Geometry: final body of the model. Coordinates: model frame, mm. Face numbers are marked on the shaded views. A direction names the side the tool comes from. Give positions to 0.01 mm unless a question says otherwise; leave off trailing zeros. Loops run counter-clockwise (first coordinate to the right, second up) from the corner with the lowest first, then second, coordinate; pieces in that order, holes last. Notation, with made-up numbers: (-36, 51) -> (-22, 51) arc R12 cw to (-22, 62) -> close; hole circle Ø1 at (-23, 46). An arc over 180 degrees is marked (long way). Answer in a Markdown table with one row per item. Add a question column.
1) Section query C-C (z = -4.5). Return the cut outline in (x, y) (3 decimals), plus the area to 3 significant figures.
2) Section query D-D (y = 8). Return the cut outline in (x, z), plus the area to 3 significant figures.
3) Section query B-B (x = 51). Return the cut outline in (y, z), plus the area to 3 significant figures.
4) First-contact query: P1, Ø10, axis at y = 31.5, z = -14, coming from the +X side; P2, Ø5, axis at y = 43, z = 10.5, coming from the -X side; P3, Ø8, axis at y = 15.5, z = -6, coming from the +X side. Flat tips, straight axial feed; report the tip coordinate or a pass-through.
5) Access query for the marked faces 5 and 6. Directions: +Z, -Z, +X, -X, +Y, -Y. A direction counts if a zero-diameter tool reaches every point of the face in a straight line with its end or side. Return the directions, or none.
6) Line query: line 1 (Y direction, x = 61.5, z = -8); line 2 (Y direction, x = 9.5, z = -15.5); line 3 (Y direction, x = 36, z = 16). Output: solid intervals per line, ascending. Write a range as from..to.
7) Section query A-A (z = 8). Return the cut outline in (x, y) (3 decimals), plus the area to 3 significant figures.
8) Draft query along Z for the marked faces 1, 2, 3 and 4. Return one class per face: +Z half, -Z half, draft (parallel to the pull), parting line (faces both ways), or undercut.
```python
from build123d import *

# Parameters (mm, degrees)
EXTRUDE_THIN1_DEPTH = 20.6375
SKETCH2_R           = 7.14375
CUT_EXTRUDE1_DEPTH  = 6.35
SKETCH3_R           = 7.14375
CUT_EXTRUDE2_DEPTH  = 6.35


with BuildPart() as part:
    # Sketch1 → Extrude-Thin1 (new, symmetric)
    with BuildSketch(Plane.XY):
        with BuildLine():
            Line((63.5, 0), (9.525, 0))
            ThreePointArc((9.525, 0), (0.725047453, 5.879940307), (2.789807909, 16.260192091))
            Line((2.789807909, 16.260192091), (52.181216575, 65.651600757))
            Line((52.181216575, 65.651600757), (56.671344636, 61.161472696))
            Line((56.671344636, 61.161472696), (7.27993597, 11.77006403))
            ThreePointArc((7.27993597, 11.77006403), (6.591682484, 8.309980102), (9.525, 6.35))
            Line((9.525, 6.35), (63.5, 6.35))
            Line((63.5, 6.35), (63.5, 0))
        make_face()
    extrude(amount=EXTRUDE_THIN1_DEPTH, both=True)

    # Sketch2 → Cut-Extrude1 (cut)
    with BuildSketch(Plane.XZ):
        with Locations((42.8625, 0)):
            Circle(SKETCH2_R)
    extrude(amount=-CUT_EXTRUDE1_DEPTH, mode=Mode.SUBTRACT)

    # Sketch3 → Cut-Extrude2 (cut)
    with BuildSketch(Plane(origin=(-6.735192091, 6.735192091, 0), x_dir=(0, 0, 1), z_dir=(-0.7071067811865439, 0.7071067811865511, 0))):
        with Locations(Location((0, 62.682884182, 0), (0, 0, 270))):
            Circle(SKETCH3_R)
    extrude(amount=-CUT_EXTRUDE2_DEPTH, mode=Mode.SUBTRACT)


solid = part.part
```
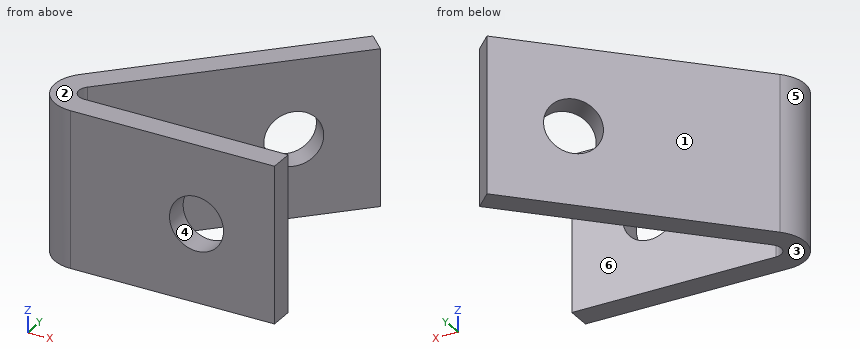
Evaluation:
| question | item | result |
|---|---|---|
| 1 | outline | (2.79, 16.26) arc R9.525 ccw to (9.525, 0) -> (37.314, 0) -> (37.314, 6.35) -> (9.525, 6.35) arc R3.175 cw to (7.28, 11.77) -> (38.155, 42.645) -> (33.665, 47.135) -> close; (41.512, 54.982) -> (46.002, 50.492) -> (56.671, 61.161) -> (52.181, 65.652) -> close; (48.411, 0) -> (63.5, 0) -> (63.5, 6.35) -> (48.411, 6.35) -> close |
| 1 | area | 740 mm² |
| 2 | outline | (0.12, -20.64) -> (6.74, -20.64) -> (6.74, 20.64) -> (0.12, 20.64) -> close |
| 2 | area | 273 mm² |
| 3 | outline | (0, -20.64) -> (6.35, -20.64) -> (6.35, 20.64) -> (0, 20.64) -> close; (55.49, -20.64) -> (64.47, -20.64) -> (64.47, 20.64) -> (55.49, 20.64) -> close |
| 3 | area | 633 mm² |
| 4 | P1 | x = 32.01 |
| 4 | P2 | x = 27.03 |
| 4 | P3 | x = 15.01 |
| 5 | face 5 | +Z, -Z, -X |
| 5 | face 6 | +Z, -Z, +X |
| 6 | line 1 | 0..6.35 |
| 6 | line 2 | 0..6.35, 13.99..22.97 |
| 6 | line 3 | 0..6.35, 40.49..49.47 |
| 7 | outline | (2.79, 16.26) arc R9.525 ccw to (9.525, 0) -> (63.5, 0) -> (63.5, 6.35) -> (9.525, 6.35) arc R3.175 cw to (7.28, 11.77) -> (56.671, 61.161) -> (52.181, 65.652) -> close |
| 7 | area | 881 mm² |
| 8 | face 1 | draft |
| 8 | face 2 | +Z half |
| 8 | face 3 | -Z half |
| 8 | face 4 | undercut |
